from build123d import *

# Parameters (mm, degrees)
SKETCH1_W             = 152.4
SKETCH1_H             = 73.025
BOSS_EXTRUDE1_DEPTH   = 6.35
SKETCH2_W             = 3.175
SKETCH2_H             = 3.175
BOSS_EXTRUDE2_DEPTH   = 9.652
SKETCH3_W             = 3.175
SKETCH3_H             = 3.175
BOSS_EXTRUDE3_DEPTH   = 3.048
M2_CLEARANCE_HOLE1_D  = 2.4
FILLET1_RADIUS        = 1.5875
FILLET1_LENGTH        = 3.175
FILLET2_R             = 1.5875
FILLET3_R             = 1.5875
FILLET4_RADIUS        = 1.5875
FILLET4_LENGTH        = 3.175
FILLET5_R             = 12.7
SKETCH9_W             = 44.45
SKETCH9_H             = 4.7625
SKETCH9_W_2           = 25.4
SKETCH9_W_3           = 9.525
SKETCH9_H_2           = 25.4
CUT_EXTRUDE1_DEPTH    = 86.998061956
F_4_CLEARANCE_HOLE1_D = 3.2639
SKETCH12_R            = 3.175
BOSS_EXTRUDE4_DEPTH   = 1.5875
F_4_CLEARANCE_HOLE3_D = 3.2639


with BuildPart() as part:
    # Sketch1 → Boss-Extrude1 (new body)
    with BuildSketch(Plane(origin=(0, 0, 0), x_dir=(1, 0, 0), z_dir=(0, 1, 0))):
        Rectangle(SKETCH1_W, SKETCH1_H)
    extrude(amount=BOSS_EXTRUDE1_DEPTH)

    # Sketch2 → Boss-Extrude2 (add)
    with BuildSketch(Plane.XZ):
        with Locations((-65.521407591, -26.442756121)):
            Rectangle(SKETCH2_W, SKETCH2_H)
    boss_extrude2 = extrude(amount=BOSS_EXTRUDE2_DEPTH)

    # Sketch3 → Boss-Extrude3 (add)
    with BuildSketch(Plane.XY.offset(-24.855256121)):
        with Locations((-65.521407591, -8.0645)):
            Rectangle(SKETCH3_W, SKETCH3_H)
    boss_extrude3 = extrude(amount=BOSS_EXTRUDE3_DEPTH)

    # Mirror1: Boss-Extrude2, Boss-Extrude3 across plane
    add(boss_extrude2.mirror(Plane.XY))
    add(boss_extrude3.mirror(Plane.XY))

    # M2 Clearance Hole1 (through all)
    with Locations(Plane(origin=(0, 0, 0), x_dir=(-1, 0, 0), z_dir=(0, -1, 0))):
        with Locations((65.0875, 31.75)):
            m2_clearance_hole1 = Hole(M2_CLEARANCE_HOLE1_D / 2)

    # Fillet1: full round fillet: the end face becomes a half cylinder, R = half its width
    fillet1_face = Plane((-65.521407591, -8.0645, 21.807256121), x_dir=(-1, 0, 0), z_dir=(0, 0, -1))  # on the end face: x along it, z out of the body
    fillet1_slab = fillet1_face.offset(-FILLET1_RADIUS / 2) * Box(FILLET1_LENGTH, 2 * FILLET1_RADIUS, FILLET1_RADIUS, mode=Mode.PRIVATE)  # the body's end, R deep
    fillet1_round = Plane((-65.521407591, -8.0645, 23.394756121), x_dir=(0, 0, -1), z_dir=(-1, 0, 0)) * Cylinder(FILLET1_RADIUS, FILLET1_LENGTH, mode=Mode.PRIVATE)  # its axis R under the face
    add(fillet1_slab - fillet1_round, mode=Mode.SUBTRACT)

    # Fillet2
    fillet2_edges = [part.edges().sort_by_distance(p)[0] for p in [
        (-65.521407591, -9.652, 28.030256121),
    ]]
    fillet(fillet2_edges, radius=FILLET2_R)

    # Mirror2: M2 Clearance Hole1 across plane
    add(m2_clearance_hole1.mirror(Plane.XY), mode=Mode.SUBTRACT)

    # Fillet3
    fillet3_edges = [part.edges().sort_by_distance(p)[0] for p in [
        (-65.521407591, -9.652, -28.030256121),
    ]]
    fillet(fillet3_edges, radius=FILLET3_R)

    # Fillet4: full round fillet: the end face becomes a half cylinder, R = half its width
    fillet4_face = Plane((-65.521407591, -8.0645, -21.807256121), x_dir=(-1, 0, 0), z_dir=(0, 0, 1))  # on the end face: x along it, z out of the body
    fillet4_slab = fillet4_face.offset(-FILLET4_RADIUS / 2) * Box(FILLET4_LENGTH, 2 * FILLET4_RADIUS, FILLET4_RADIUS, mode=Mode.PRIVATE)  # the body's end, R deep
    fillet4_round = Plane((-65.521407591, -8.0645, -23.394756121), x_dir=(0, 0, 1), z_dir=(-1, 0, 0)) * Cylinder(FILLET4_RADIUS, FILLET4_LENGTH, mode=Mode.PRIVATE)  # its axis R under the face
    add(fillet4_slab - fillet4_round, mode=Mode.SUBTRACT)

    # Fillet5
    fillet5_edges = [part.edges().sort_by_distance(p)[0] for p in [
        (76.2, 3.175, 36.5125),
        (-76.2, 3.175, 36.5125),
        (-76.2, 3.175, -36.5125),
        (76.2, 3.175, -36.5125),
    ]]
    fillet(fillet5_edges, radius=FILLET5_R)

    # Sketch9 → Cut-Extrude1 (cut, through all)
    with BuildSketch(Plane(origin=(0, 6.35, 0), x_dir=(1, 0, 0), z_dir=(0, 1, 0))):
        with Locations((-47.625, -8.73125)):
            Rectangle(SKETCH9_W, SKETCH9_H)
        with Locations((-47.625, 8.73125)):
            Rectangle(SKETCH9_W_2, SKETCH9_H)
        Rectangle(SKETCH9_W_3, SKETCH9_H_2)
    extrude(amount=-CUT_EXTRUDE1_DEPTH, mode=Mode.SUBTRACT)

    # #4 Clearance Hole1 (through all)
    with Locations(Plane(origin=(0, 6.35, 0), x_dir=(1, 0, 0), z_dir=(0, 1, 0))):
        with Locations((-65.88125, 7.9375), (-29.36875, 7.9375)):
            Hole(F_4_CLEARANCE_HOLE1_D / 2)

    # Sketch12 → Boss-Extrude4 (add)
    with BuildSketch(Plane(origin=(0, 6.35, 0), x_dir=(1, 0, 0), z_dir=(0, 1, 0))):
        with Locations(Location((9.525, 28.575, 0), (0, 0, 270))):
            Circle(SKETCH12_R)
        with Locations(Location((41.275, 28.575, 0), (0, 0, 270))):
            Circle(SKETCH12_R)
        with Locations(Location((41.275, 6.35, 0), (0, 0, 270))):
            Circle(SKETCH12_R)
        with Locations(Location((9.525, 6.35, 0), (0, 0, 270))):
            Circle(SKETCH12_R)
        with Locations(Location((11.1125, -6.35, 0), (0, 0, 270))):
            Circle(SKETCH12_R)
        with Locations(Location((11.1125, -26.9875, 0), (0, 0, 270))):
            Circle(SKETCH12_R)
        with Locations(Location((71.4375, -26.9875, 0), (0, 0, 270))):
            Circle(SKETCH12_R)
        with Locations(Location((71.4375, -6.35, 0), (0, 0, 270))):
            Circle(SKETCH12_R)
    extrude(amount=BOSS_EXTRUDE4_DEPTH)

    # #4 Clearance Hole3 (through all)
    with Locations(Plane(origin=(0, 7.9375, 0), x_dir=(1, 0, 0), z_dir=(0, 1, 0))):
        with Locations((9.525, 28.575), (41.275, 28.575), (41.275, 6.35), (9.525, 6.35), (11.1125, -6.35), (11.1125, -26.9875), (71.4375, -26.9875), (71.4375, -6.35)):
            Hole(F_4_CLEARANCE_HOLE3_D / 2)


solid = part.part
The listing builds one solid part. Answer for the finished solid, in the listing's coordinates (mm). A direction names the side the tool comes from. Coordinates: 2 decimals unless noted, no trailing zeros. Loops run counter-clockwise (first coordinate to the right, second up) from the corner with the lowest first, then second, coordinate; pieces in that order, holes last. Notation, with made-up numbers: (49.25, 3.5) -> (73.25, 3.5) arc R25 ccw to (73.25, 39.5) -> close; hole circle Ø3 at (35.5, 5.25). An arc over 180 degrees is marked (long way). Write item = value, one per line. Start each with the question number.
1) The mould has two halves that part along X. Classify faces 1 (the face through (72.58, 3.22, 32.69)), 2 (the face through (-60.325, 3, -9)), 3 (the face through (-66, -3, -24.855)), 4 (the face through (-48, 3, -6.35)): released by +X, released by -X, zero draft, split by the parting line, or undercut.
2) A cutting plane is placed at C-C (z = 16). Give the vertices of the cut face in (x, y), then the cut area to 3 significant figures.
3) A cutting plane is placed at A-A (y = -4.75). Give the vertices of the cut face in (x, z), then the cut area to 3 significant figures.
4) Straight lines are drawn through the part: line 1 (Z direction, x = 0, y = 3); line 2 (X direction, y = 3.75, z = 6.5); line 3 (Y direction, x = 29, z = -10). For each, find the intervals that lie inside material, in ascending order. Write a range as from..to.
5) Given pin 1 Ø1 at (x, z) = (51, -5.5) entering from +Y; pin 2 Ø1 at (x, z) = (-5, -22) entering from -Y; pin 3 Ø10 at (x, y) = (-45.5, -4) entering from -Z; pin 4 Ø7 at (y, z) = (-6, -24.5) entering from -X, each flat-ended and moving along its own axis, determine where each tip first touches the part or whether it passes through.
6) A cutting plane is placed at B-B (x = 16.5). Give the vertices of the cut face in (y, z), then the cut area to 3 significant figures.
7) A tool of negligible diameter and unlimited length cuts with its end or side. For faces 5 (the face through (74.585, 7.133, 5.937)), 6 (the face through (-66, -4, -28.03)), 7 (the face through (-4.762, 3, 0)), from which of +Z, -Z, +X, -X, +Y, -Y can it reach the whole face along a straight path? Write none if from no direction.
Responses:
q1.face_1 = released by +X
q1.face_2 = undercut
q1.face_3 = zero draft
q1.face_4 = undercut
q2.outline = (-76.2, 0) -> (76.2, 0) -> (76.2, 6.35) -> (-76.2, 6.35) -> close
q2.area = 968 mm²
q3.outline = (-67.11, -28.03) -> (-63.93, -28.03) -> (-63.93, -24.86) -> (-67.11, -24.86) -> close; (-67.11, 24.86) -> (-63.93, 24.86) -> (-63.93, 28.03) -> (-67.11, 28.03) -> close
q3.area = 20.2 mm²
q4.line_1 = -36.51..-12.7, 12.7..36.51
q4.line_2 = -76.2..-69.85, -25.4..-4.76, 4.76..9.49, 12.74..69.81, 73.06..76.2
q4.line_3 = 0..6.35
q5.pin_1 = 6.35
q5.pin_2 = 0
q5.pin_3 = -36.51
q5.pin_4 = -67.11
q6.outline = (0, -36.51) -> (6.35, -36.51) -> (6.35, 36.51) -> (0, 36.51) -> close
q6.area = 464 mm²
q7.face_5 = +Y
q7.face_6 = -Z, +X, -X, -Y
q7.face_7 = +Y, -Y
